For this review, take the finished solid that the model builds, in its own axes (mm). Face numbers are marked on the shaded views. A direction names the side the tool comes from. Coordinates: 2 decimals unless noted, no trailing zeros. Write each loop counter-clockwise with the first axis right and the second up, starting at its lowest first coordinate (ties: lowest second). Pieces come first, ordered by that corner, then holes. Notation, with made-up numbers: M 30.5,83.25 L 85.5,83.25 A18 ccw 85.5,104.25 Z; hole C 53,-36 d1. An arc over 180 degrees is marked long. Return JSON: item names as keys, results as strings.
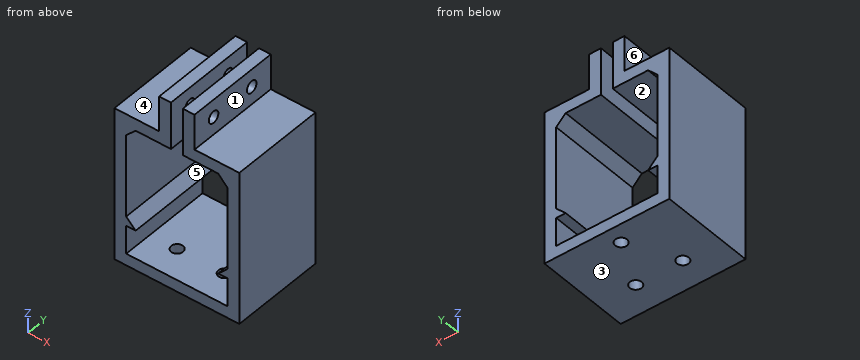
```python
from build123d import *

# Parameters (mm, degrees)
MAIN_DEPTH          = 40
CHAMFER_1_SIZE      = 4
HOLES_REACH         = 105.966
SKETCH_2_R          = 2.5
EXTRUDE_3_DEPTH     = 40
CUT_EXTRUDE_4_REACH = 85.552
SKETCH_4_R          = 2.5


with BuildPart() as part:
    # Эскиз1 → main (new body)
    with BuildSketch(Plane(origin=(0, 0, 0), x_dir=(1, 0, 0), z_dir=(0, 1, 0))):
        Polygon((0, 0), (0, 65), (53, 65), (53, 0), (34, 0), (34, -15), (29, -15), (29, 5), (48, 5), (48, 60), (5, 60), (5, 5), (24, 5), (24, -15), (19, -15), (19, 0), align=None)
    extrude(amount=MAIN_DEPTH)

    # Фаска1
    chamfer_1_edges = [part.edges().sort_by_distance(p)[0] for p in [
        (48, 20, -5),
        (5, 20, -5),
    ]]
    chamfer(chamfer_1_edges, length=CHAMFER_1_SIZE)

    # Эскиз2 → holes (cut, up to next)
    with BuildSketch(Plane(origin=(0, 0, -65), x_dir=(-1, 0, 0), z_dir=(0, 0, -1)), mode=Mode.PRIVATE) as holes_sk1:
        with Locations((-26.5, 32.5)):
            Circle(SKETCH_2_R)
    holes_tool1 = extrude(holes_sk1.sketch, amount=-HOLES_REACH, mode=Mode.PRIVATE) & part.part
    # Эскиз2 → holes (cut, up to next)
    with BuildSketch(Plane(origin=(0, 0, -65), x_dir=(-1, 0, 0), z_dir=(0, 0, -1)), mode=Mode.PRIVATE) as holes_sk2:
        with Locations((-36.5, 12.5)):
            Circle(SKETCH_2_R)
    holes_tool2 = extrude(holes_sk2.sketch, amount=-HOLES_REACH, mode=Mode.PRIVATE) & part.part
    # Эскиз2 → holes (cut, up to next)
    with BuildSketch(Plane(origin=(0, 0, -65), x_dir=(-1, 0, 0), z_dir=(0, 0, -1)), mode=Mode.PRIVATE) as holes_sk3:
        with Locations((-16.5, 12.5)):
            Circle(SKETCH_2_R)
    holes_tool3 = extrude(holes_sk3.sketch, amount=-HOLES_REACH, mode=Mode.PRIVATE) & part.part
    add(holes_tool1.solids().sort_by_distance((26.5, 32.5, -65))[0], mode=Mode.SUBTRACT)
    add(holes_tool2.solids().sort_by_distance((36.5, 12.5, -65))[0], mode=Mode.SUBTRACT)
    add(holes_tool3.solids().sort_by_distance((16.5, 12.5, -65))[0], mode=Mode.SUBTRACT)

    # Эскиз3 → Вытянуть3 (add)
    with BuildSketch(Plane(origin=(0, 0, 0), x_dir=(1, 0, 0), z_dir=(0, 1, 0))):
        Polygon((5, 44), (5, 48), (9, 48), align=None)
        Polygon((44, 48), (48, 44), (48, 48), align=None)
    extrude(amount=EXTRUDE_3_DEPTH)

    # Вытянуть4: up to this face of the body (flat: up to its plane)
    cut_extrude_4_end = Plane(part.part.faces().sort_by_distance((19, 20, 7.5))[0])
    # Эскиз4 → Вытянуть4 (cut, up to the picked face)
    with BuildSketch(Plane(origin=(34, 0, 0), x_dir=(0, 0, -1), z_dir=(1, 0, 0)), mode=Mode.PRIVATE) as cut_extrude_4_sk1:
        with Locations((-7.5, 10)):
            Circle(SKETCH_4_R)
    cut_extrude_4_tool1 = split(extrude(cut_extrude_4_sk1.sketch, amount=-CUT_EXTRUDE_4_REACH, mode=Mode.PRIVATE), bisect_by=cut_extrude_4_end, keep=Keep.BOTH, mode=Mode.PRIVATE)
    # Эскиз4 → Вытянуть4 (cut, up to the picked face)
    with BuildSketch(Plane(origin=(34, 0, 0), x_dir=(0, 0, -1), z_dir=(1, 0, 0)), mode=Mode.PRIVATE) as cut_extrude_4_sk2:
        with Locations((-7.5, 30)):
            Circle(SKETCH_4_R)
    cut_extrude_4_tool2 = split(extrude(cut_extrude_4_sk2.sketch, amount=-CUT_EXTRUDE_4_REACH, mode=Mode.PRIVATE), bisect_by=cut_extrude_4_end, keep=Keep.BOTH, mode=Mode.PRIVATE)
    add(cut_extrude_4_tool1.solids().sort_by(Axis((34, 10, 7.5), (-1, 0, 0)))[0], mode=Mode.SUBTRACT)
    add(cut_extrude_4_tool2.solids().sort_by(Axis((34, 30, 7.5), (-1, 0, 0)))[0], mode=Mode.SUBTRACT)


solid = part.part
```
1. We need section B-B (z = 7.5). State the section outline as (x, y) points.
Checks:
{"outline": "M 19,0 L 24,0 L 24,7.5 L 19,7.5 Z; M 19,12.5 L 24,12.5 L 24,27.5 L 19,27.5 Z; M 19,32.5 L 24,32.5 L 24,40 L 19,40 Z; M 29,0 L 34,0 L 34,7.5 L 29,7.5 Z; M 29,12.5 L 34,12.5 L 34,27.5 L 29,27.5 Z; M 29,32.5 L 34,32.5 L 34,40 L 29,40 Z"}
2. Clearance check with flat-ended pins moving along their axes: pin 1 Ø3 at (x, y) = (16.5, 12.5) entering from +Z; pin 2 Ø4.5 at (y, z) = (18, 6) entering from -X; pin 3 Ø1 at (y, z) = (10.5, 3.5) entering from +X. State where each tip first meets the part, or that it passes through.
Checks:
{"pin 1": "z = 0", "pin 2": "x = 19", "pin 3": "x = 34"}
3. Draft analysis for pull direction Z (two halves, no side actions). For the marked faces 4, 5 and 6, state which applies: +Z half, -Z half, draft (parallel to the pull), parting line (faces both ways), or undercut.
Checks:
{"face 4": "+Z half", "face 5": "undercut", "face 6": "draft"}
4. We need section A-A (x = 41.5). State the section outline as (y, z) points.
Checks:
{"outline": "M 0,-65 L 40,-65 L 40,-60 L 0,-60 Z; M 0,-5 L 40,-5 L 40,0 L 0,0 Z"}
5. For the marked faces 1, 2 and 3, list the 3-axis set-ups (+Z, -Z, +X, -X, +Y, -Y) from which the entire face can be reached by the end or side of a thin tool; tool diameter is ignored.
Checks:
{"face 1": "+Z, +X, +Y, -Y", "face 2": "+Y, -Y", "face 3": "-Z, +X, -X, +Y, -Y"}
6. We need section D-D (x = 16.5). State the section outline as (y, z) points.
Checks:
{"outline": "M 0,-65 L 10,-65 L 10,-60 L 0,-60 Z; M 0,-5 L 40,-5 L 40,0 L 0,0 Z; M 15,-65 L 40,-65 L 40,-60 L 15,-60 Z"}
7. We need section C-C (z = -29.5). State the section outline as (x, y) points, plus the area to 3 significant figures.
Checks:
{"outline": "M 0,0 L 5,0 L 5,40 L 0,40 Z; M 48,0 L 53,0 L 53,40 L 48,40 Z", "area": "400 mm2"}
8. Wall thickness on L1, parallel to Y at x = 30.45, z = 7.5; L2, parallel to X at y = 37, z = -44; L3, parallel to Z at x = 21, y = 6: over which ranges is each line inside the solid? List them lowest first. Write a range as from..to.
Checks:
{"L1": "0..7.5, 12.5..27.5, 32.5..40", "L2": "0..5, 48..53", "L3": "-65..-60, -5..15"}
